```python
from build123d import *

# Parameters (mm, degrees)
SKETCH_1_R                    = 17.5
EXTRUDE_1_DEPTH               = 5
HOLE_WIZARD_M3_1_D            = 3.4
HOLE_WIZARD_M3_1_CSINK_D      = 3.45
HOLE_WIZARD_M3_1_CSINK_ANGLE  = 90
PATTERN_CIRCULAR_1_COUNT      = 6
HOLE_WIZARD_M3_1_2_AT_2_COUNT = 2
HOLE_WIZARD_M3_1_2_AT_2_PITCH = 12


with BuildPart() as part:
    # 草图1 → 凸台-拉伸1 (new body)
    with BuildSketch(Plane(origin=(0, 0, 0), x_dir=(1, 0, 0), z_dir=(0, 1, 0))):
        with Locations(Location((0, 0, 0), (0, 0, 270))):
            Circle(SKETCH_1_R)
    extrude(amount=EXTRUDE_1_DEPTH)

    # Hole Wizard M3 _1 (through all)
    with Locations(Plane(origin=(0, 0, 0), x_dir=(-1, 0, 0), z_dir=(0, -1, 0))):
        with Locations((11.691342951, 6.75)):
            hole_wizard_m3_1 = CounterSinkHole(HOLE_WIZARD_M3_1_D / 2, HOLE_WIZARD_M3_1_CSINK_D / 2, counter_sink_angle=HOLE_WIZARD_M3_1_CSINK_ANGLE)

    # 阵列(圆周)1: Hole Wizard M3 _1 ×6 about axis, 2 skipped
    pattern_circular_1_axis = Axis((0, 0, 0), (0, -1, 0))
    add([hole_wizard_m3_1.rotate(pattern_circular_1_axis, i * 360 / PATTERN_CIRCULAR_1_COUNT) for i in range(1, PATTERN_CIRCULAR_1_COUNT) if i not in (1, 4)], mode=Mode.SUBTRACT)

    # 草图6 → Hole Wizard M3 _1 2 (revolve, cut)
    with BuildSketch(Plane(origin=(0, 5, -6), x_dir=(0, 0, 1), z_dir=(1, 0, 0))):
        Polygon((0, 0), (0, 5), (1.7, 5), (1.7, 3.5), (3, 3.5), (3, 0.025), (3.025, 0), align=None)
    hole_wizard_m3_1_2 = revolve(axis=Axis((0, 11.35, -6), (0, -1, 0)), mode=Mode.SUBTRACT)

    # Hole Wizard M3 _1 2 at 2: Hole Wizard M3 _1 2 ×2
    with Locations(*[(0, 0, i * HOLE_WIZARD_M3_1_2_AT_2_PITCH) for i in range(1, HOLE_WIZARD_M3_1_2_AT_2_COUNT)]):
        add(hole_wizard_m3_1_2, mode=Mode.SUBTRACT)


solid = part.part
```
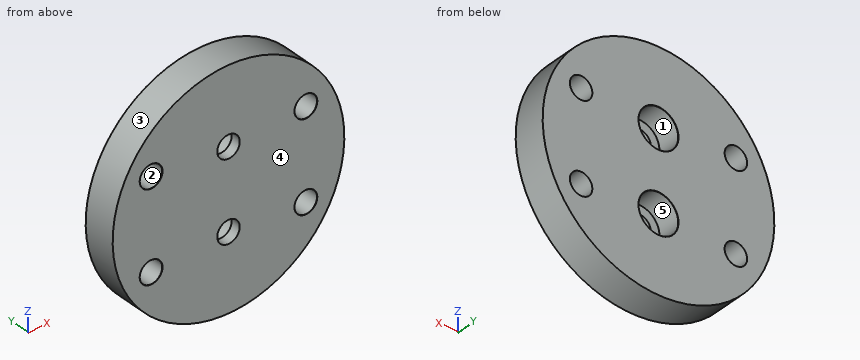
Read the model definition and answer for the solid it produces. Units are mm, in the model's axes. Face numbers are marked on the shaded views. A direction names the side the tool comes from. Round coordinates to 2 decimals unless told otherwise and drop trailing zeros. Write each loop counter-clockwise with the first axis right and the second up, starting at its lowest first coordinate (ties: lowest second). Pieces come first, ordered by that corner, then holes. Notation, with made-up numbers: (82.5, 35.25) - (115.5, 35.25) arc R9 cw to (115.5, 51.25) - close; hole circle Ø4 at (76.5, 35.25). An arc over 180 degrees is marked (long way). Use CSV: the item, a comma, the result in double quotes.
Q1. Each of these flat-tipped pins is pushed along its axis until it touches: pin 1 Ø2 at (y, z) = (4.5, 4) entering from -X; pin 2 Ø1.5 at (x, y) = (-13, 1.5) entering from -Z. Where does it stop, or does it pass through?
Values:
pin 1,"stops at x = -17.24"
pin 2,"stops at z = -12.5"
Q2. Find section A-A, the plane x = 0. Write down the section's boundary in (y, z) (3 decimals), then the cut area to 3 significant figures.
Values:
outline,"(0, -17.5) - (5, -17.5) - (5, -9.025) - (4.975, -9) - (1.5, -9) - (1.5, -7.7) - (0, -7.7) - close; (0, -4.3) - (1.5, -4.3) - (1.5, -3) - (4.975, -3) - (5, -2.975) - (5, 2.975) - (4.975, 3) - (1.5, 3) - (1.5, 4.3) - (0, 4.3) - close; (0, 7.7) - (1.5, 7.7) - (1.5, 9) - (4.975, 9) - (5, 9.025) - (5, 17.5) - (0, 17.5) - close"
area,"123 mm²"
Q3. Straight lines are drawn through the part: line 1 along X through (y, z) = (0.95, 6); line 2 along Z through (x, y) = (-1, 1.65); line 3 along Z through (x, y) = (13, 1.3). For each, find the intervals that lie inside material, in ascending order.
Values:
line 1,"x = -16.44 to -13.22, -10.17 to -1.7, 1.7 to 10.17, 13.22 to 16.44"
line 2,"z = -17.47 to -8.83, -3.17 to 3.17, 8.83 to 17.47"
line 3,"z = -11.72 to -7.84, -5.66 to 5.66, 7.84 to 11.72"
Q4. Determine the mould class of the marked faces 3, 4 and 5 for opening direction X: +X half, -X half, draft (parallel to the pull), parting line (faces both ways), or undercut.
Values:
face 3,"parting line"
face 4,"draft"
face 5,"undercut"
Q5. A tool of negligible diameter and unlimited length cuts with its end or side. For the marked faces 1 and 2, from which of +Z, -Z, +X, -X, +Y, -Y can it reach the whole face along a straight path? Write none if from no direction.
Values:
face 1,"+Y"
face 2,"+Y, -Y"
Q6. Find section C-C, the plane z = -9.5. Write down the section's boundary in (x, y), then the cut area to 3 significant figures.
Values:
outline,"(-14.7, 0) - (14.7, 0) - (14.7, 5) - (-14.7, 5) - close"
area,"147 mm²"
Q7. Find section B-B, the plane y = 2.55. Write down the section's boundary in (x, z), then the cut area to 3 significant figures.
Values:
outline,"circle Ø35 at (0, 0); hole circle Ø3.4 at (-11.69, -6.75); hole circle Ø3.4 at (-11.69, 6.75); hole circle Ø6 at (0, -6); hole circle Ø6 at (0, 6); hole circle Ø3.4 at (11.69, -6.75); hole circle Ø3.4 at (11.69, 6.75)"
area,"869 mm²"
Q8. Find section D-D, the plane z = 6.75. Count the separate pieces of the cut face and the enclosed holes in it, then the cut area to 3 significant figures.
Values:
separate pieces,"4"
enclosed holes,"0"
area,"103 mm²"
